Autodesk Inventor part; units mm, degrees
ref_plane "YZ Plane" through (0, 0, 0) normal (1, 0, 0) x (0, 1, 0)
ref_plane "XZ Plane" through (0, 0, 0) normal (0, 1, 0) x (-1, 0, 0)
ref_plane "XY Plane" through (0, 0, 0) normal (0, 0, 1) x (1, 0, 0)
sketch "スケッチ1" plane through (0, 0, 0) normal (0, 0, 1) x (1, 0, 0)
  line L0 (10, -10) -> (-10, -10)
  line L1 (-10, -10) -> (-10, 10)
  line L2 (-10, 10) -> (10, 10)
  line L3 (10, 10) -> (10, -10)
  line L4 (10, -10) -> (-10, 10) construction
  line L5 (-10, -10) -> (10, 10) construction
  line L6 (8, 8) -> (-8, 8)
  line L7 (-8, 8) -> (-8, -8)
  line L8 (-8, -8) -> (8, -8)
  line L9 (8, -8) -> (8, 8)
  point P0 (0, 0)
  dimension "d0" = 20
  dimension "d1" = 20
  dimension "d2" = 2
extrude "押し出し1" add sketch "スケッチ1" along normal blind 360
sketch "スケッチ2" plane through (-10, 10, 0) normal (0, 1, 0) x (1, 0, 0)
  line L0 (10, 0) -> (10, -360)
  line L1 (2, -360) -> (18, -360)
  line L2 (20, 0) -> (0, 0)
  point P0 (10, -350)
  point P1 (10, -300)
  point P2 (10, -60)
  point P3 (10, -10)
  dimension "d5" = 10
  dimension "d6" = 50
  dimension "d7" = 50
  dimension "d9" = 10
hole "穴1" at (0, 10, 350) at (0, 10, 300) at (0, 10, 60) at (0, 10, 10) direction (0, -1, 0) diameter 4 end through all
sketch "スケッチ3" plane through (10, -10, 0) normal (1, 0, 0) x (0, 0, -1)
  line L0 (0, 10) -> (-360, 10)
  line L1 (-360, 20) -> (-360, 0)
  line L2 (0, 0) -> (0, 20)
  point P0 (-340, 10)
  point P1 (-290, 10)
  point P2 (-20, 10)
  point P3 (-70, 10)
  dimension "d17" = 20
  dimension "d18" = 50
  dimension "d19" = 20
  dimension "d20" = 50
hole "穴2" at (10, 0, 340) at (10, 0, 290) at (10, 0, 20) at (10, 0, 70) direction (-1, 0, 0) diameter 3.3 end through all
properties part number "small_kaku_2020_tka"
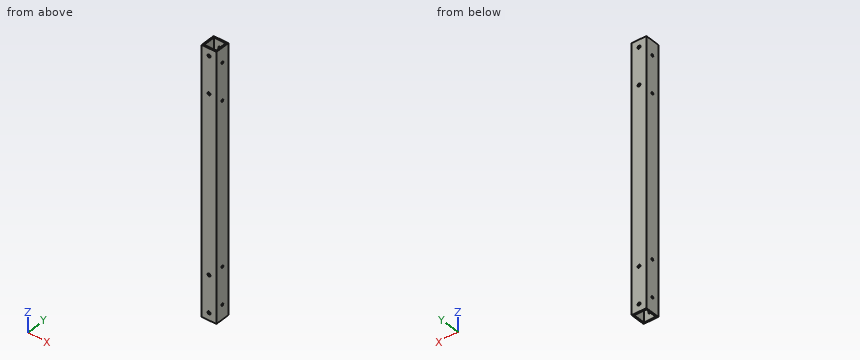
Read the model definition and answer for the solid it produces. Units are mm, in the model's axes. Give positions to 0.01 mm unless a question says otherwise; leave off trailing zeros. Order: outer loops, then holes, each group sorted by start corner. A loop starts at its lowest first (then second) coordinate and runs counter-clockwise, first axis right, second up.
(1) Given pin 1 (3.5 mm diameter, centred on x = 0, z = 300, fed in from -Y), flat-ended and moving along its own axis, determine where the tip first touches the part or whether it passes through.
(2) Straight lines are drawn through the part: L1, parallel to Z at x = -8.45, y = 0; L2, parallel to Z at x = 0, y = 8.6; L3, parallel to X at y = -8.4, z = 60. For each, find the intervals that lie inside material, in ascending order.
(3) Find section A-A (z = 225). Give the vertices of the cut face in (x, y).
Result sheet:
1. pin 1: passes through
2. L1: z = 0 to 18.35, 21.65 to 68.35, 71.65 to 288.35, 291.65 to 338.35, 341.65 to 360
2. L2: z = 0 to 8, 12 to 58, 62 to 298, 302 to 348, 352 to 360
2. L3: x = -10 to -2, 2 to 10
3. outline: (-10, -10) - (10, -10) - (10, 10) - (-10, 10) - close; hole (-8, -8) - (8, -8) - (8, 8) - (-8, 8) - close
